Answer from the drawing. Dimensions are ordinates in mm from the lowest x, y and z of the part. A direction names the side the tool comes from. Round coordinates to 2 decimals unless told otherwise and drop trailing zeros. Write each loop counter-clockwise with the first axis right and the second up, starting at its lowest first coordinate (ties: lowest second). Pieces come first, ordered by that corner, then holes. Notation, with made-up numbers: (-29.5, -6) - (10.5, -6) arc R25 ccw to (10.5, 8) - close; hole circle Ø3 at (-12.5, 37.5). An arc over 180 degrees is marked (long way). Answer as a JSON object with one key per item and string values.
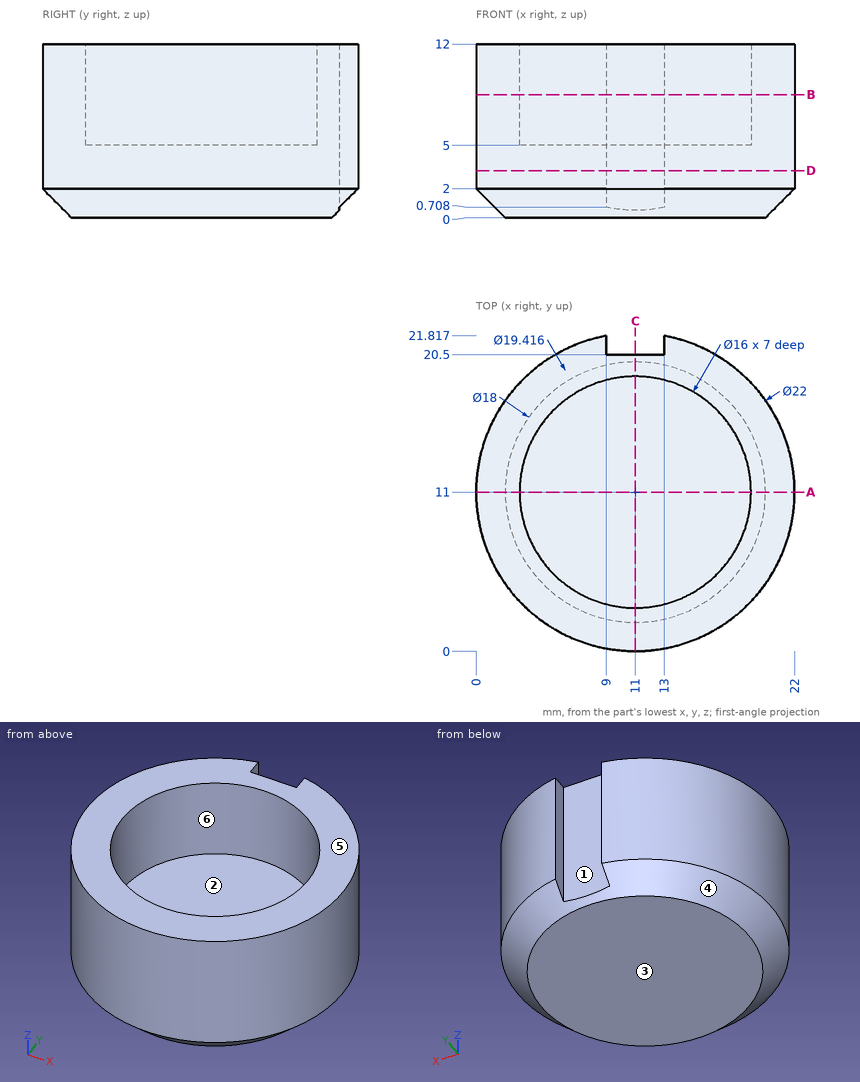
Item 1: Determine the mould class of the marked faces 4, 5 and 6 for opening direction X: pulls with the +X half, pulls with the -X half, needs draft (parallel to the pull), parting line crosses it, or undercut.
Results found:
{"face 4": "parting line crosses it", "face 5": "needs draft", "face 6": "undercut"}
Item 2: Each of these flat-tipped pins is pushed along its axis until it touches: P1, Ø5, axis at x = 10, y = 9, coming from the +Z side; P2, Ø0.7, axis at y = 21, z = 7.5, coming from the -X side; P3, Ø1, axis at y = 3.5, z = 5, coming from the -X side (1 decimal). Where does it stop, or does it pass through?
Results found:
{"P1": "z = 5", "P2": "x = 5.72", "P3": "x = 2.5"}
Item 3: For the marked faces 1, 2 and 3, determine the directions among +Z, -Z, +X, -X, +Y, -Y from which every point of the face is accessible in a straight line to the end or side of a thin tool.
Results found:
{"face 1": "+Z, -Z, +Y", "face 2": "+Z", "face 3": "-Z, +X, -X, +Y, -Y"}
Item 4: Consider line 1 along Y through (x, z) = (11, 8); line 2 along Z through (x, y) = (13.5, 16.75); line 3 along Y through (x, z) = (4, 11) (1 decimal). Determine where each line is inside the solid, lowest interval first.
Results found:
{"line 1": "0 to 3, 19 to 20.5", "line 2": "0 to 5", "line 3": "2.5 to 7.1, 14.9 to 19.5"}
Item 5: A cutting plane is placed at D-D (z = 3.25). Write down the section's boundary in (x, y).
Results found:
{"outline": "(9, 20.5) - (9, 21.82) arc R11 ccw (long way) to (13, 21.82) - (13, 20.5) - close"}
Item 6: A cutting plane is placed at A-A (y = 11). Write down the section's boundary in (x, z), and give its area (3 significant figures).
Results found:
{"outline": "(0, 2) - (2, 0) - (20, 0) - (22, 2) - (22, 12) - (19, 12) - (19, 5) - (3, 5) - (3, 12) - (0, 12) - close", "area": "148 mm²"}
Item 7: A cutting plane is placed at B-B (z = 8.5). Write down the section's boundary in (x, y).
Results found:
{"outline": "(9, 20.5) - (9, 21.82) arc R11 ccw (long way) to (13, 21.82) - (13, 20.5) - close; hole circle Ø16 at (11, 11)"}
Item 8: A cutting plane is placed at C-C (x = 11). Write down the section's boundary in (y, z).
Results found:
{"outline": "(0, 2) - (2, 0) - (20, 0) - (20.5, 0.5) - (20.5, 12) - (19, 12) - (19, 5) - (3, 5) - (3, 12) - (0, 12) - close"}
